Study the drawing (mm; zero at the part's minimum x, y, z) and answer. A direction names the side the tool comes from. Give positions to 0.01 mm unless a question says otherwise; leave off trailing zeros. Loops run counter-clockwise (first coordinate to the right, second up) from the corner with the lowest first, then second, coordinate; pieces in that order, holes last. Notation, with made-up numbers: (68.25, -31) - (93.25, -31) arc R17 cw to (93.25, 0) - close; hole circle Ø8 at (31, 13). An arc over 180 degrees is marked (long way). Write item = value, one per line. Start each with the question number.
1) Flat-ended cylindrical pins translate along their axes: P1, Ø4, axis at x = 12.5, z = 48, coming from the +Y side; P2, Ø7.5, axis at x = 29.99, z = 29.67, coming from the -Y side. Find the tip coordinate at first contact, or state that the pin passes through.
2) Which of the six approach directions +Z, -Z, +X, -X, +Y, -Y give full straight-line access (tool end or side, diameter ignored) to the marked faces 4 and 5?
3) The part is cut by section C-C on y = 10.25. Write down the section's boundary in (x, z).
4) The part is cut by section A-A on z = 15. Write down the section's boundary in (x, y).
5) The part is cut by section D-D on z = 33. Write down the section's boundary in (x, y), plus the area to 3 significant figures.
6) Consider probe 1 along X at (y, z) = (1.65, 15); probe 2 along X at (y, z) = (10.25, 15). Determine where each line is inside the solid, lowest interval first.
7) The part is cut by section B-B on x = 15. Write down the section's boundary in (y, z).
8) The mould has two halves that part along Z. Classify the marked faces 1, 2 and 3: +Z half, -Z half, draft (parallel to the pull), parting line (faces both ways), or undercut.
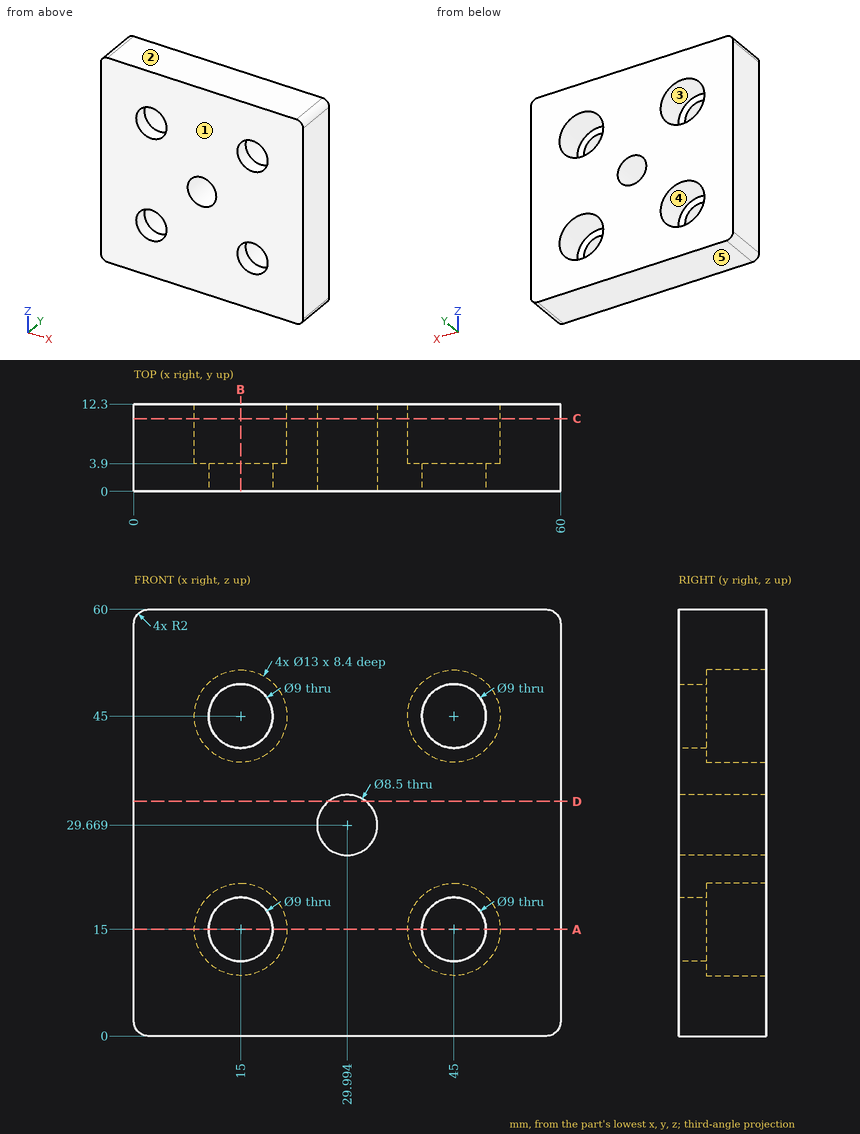
Answer below:
q1.P1 = 3.9
q1.P2 = through
q2.face_4 = +Y
q2.face_5 = -Z, +X, -X, +Y, -Y
q3.outline = (0, 2) arc R2 ccw to (2, 0) - (58, 0) arc R2 ccw to (60, 2) - (60, 58) arc R2 ccw to (58, 60) - (2, 60) arc R2 ccw to (0, 58) - close; hole circle Ø13 at (15, 15); hole circle Ø13 at (15, 45); hole circle Ø8.5 at (29.99, 29.67); hole circle Ø13 at (45, 15); hole circle Ø13 at (45, 45)
q4.outline = (0, 0) - (10.5, 0) - (10.5, 3.9) - (8.5, 3.9) - (8.5, 12.3) - (0, 12.3) - close; (19.5, 0) - (40.5, 0) - (40.5, 3.9) - (38.5, 3.9) - (38.5, 12.3) - (21.5, 12.3) - (21.5, 3.9) - (19.5, 3.9) - close; (49.5, 0) - (60, 0) - (60, 12.3) - (51.5, 12.3) - (51.5, 3.9) - (49.5, 3.9) - close
q5.outline = (0, 0) - (27.35, 0) - (27.35, 12.3) - (0, 12.3) - close; (32.63, 0) - (60, 0) - (60, 12.3) - (32.63, 12.3) - close
q5.area = 673 mm2
q6.probe_1 = 0 to 10.5, 19.5 to 40.5, 49.5 to 60
q6.probe_2 = 0 to 8.5, 21.5 to 38.5, 51.5 to 60
q7.outline = (0, 0) - (12.3, 0) - (12.3, 8.5) - (3.9, 8.5) - (3.9, 10.5) - (0, 10.5) - close; (0, 19.5) - (3.9, 19.5) - (3.9, 21.5) - (12.3, 21.5) - (12.3, 38.5) - (3.9, 38.5) - (3.9, 40.5) - (0, 40.5) - close; (0, 49.5) - (3.9, 49.5) - (3.9, 51.5) - (12.3, 51.5) - (12.3, 60) - (0, 60) - close
q8.face_1 = draft
q8.face_2 = +Z half
q8.face_3 = undercut
